Can you work these out from the drawing? Everything is in mm from the part's minimum corner. Coordinates: 2 decimals unless noted, no trailing zeros. Loops run counter-clockwise (first coordinate to the right, second up) from the corner with the lowest first, then second, coordinate; pieces in that order, holes last. Notation, with made-up numbers: M 76.5,58.5 L 102.5,58.5 A23 ccw 102.5,93.5 Z; hole C -24.75,-25 d10. An arc over 180 degrees is marked long. Write each question's results on one line, items separated by ' | '.
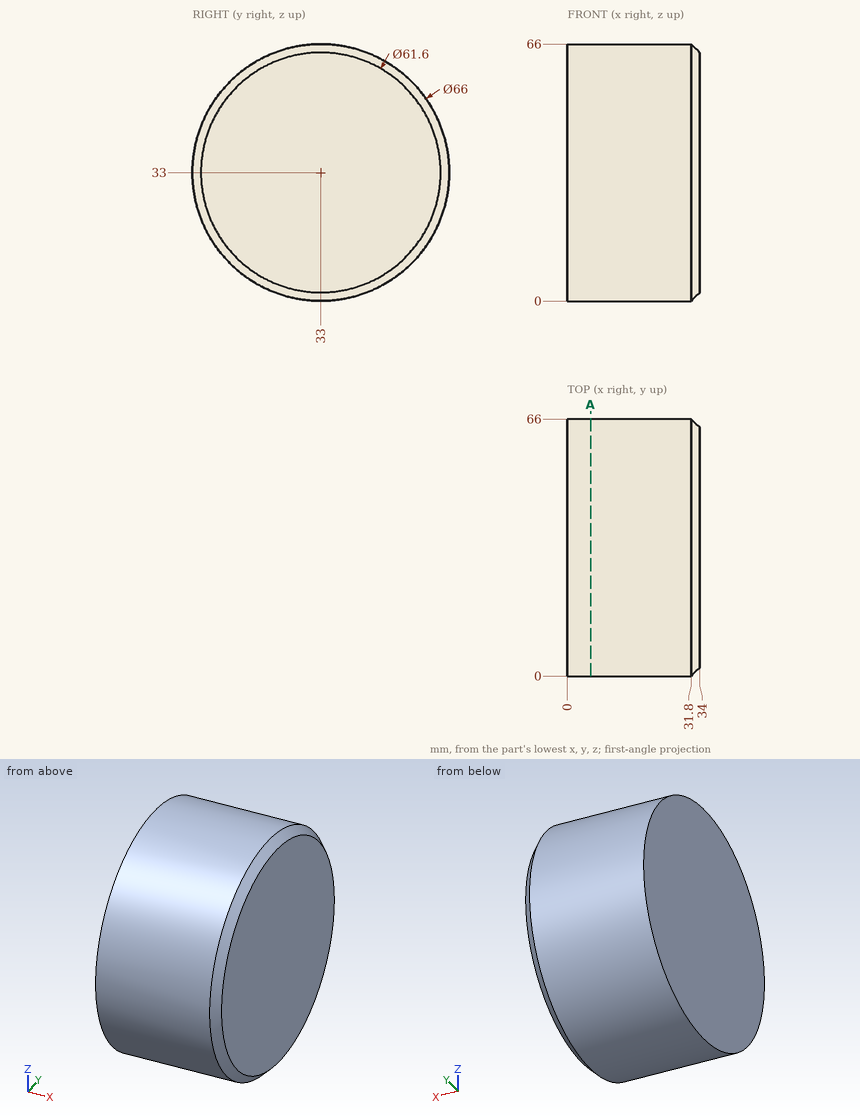
(1) Please list where these lines run through material, in increasing order: probe 1 along Z at (x, y) = (13, 34); probe 2 along Y at (x, z) = (11, 28.5). Write a range as from..to.
Reported:
probe 1: z = 0.02..65.98 | probe 2: y = 0.31..65.69
(2) Will these pins go through, and if not, where does the flat tip stop? P1, Ø10, axis at x = 9, z = 45, coming from the -Y side; P2, Ø10, axis at x = 30.5, z = 24, coming from the +Y side; P3, Ø1.5, axis at x = 22.5, y = 38.5, coming from the +Z side.
Reported:
P1: stops at y = 0.75 | P2: stops at y = 65.76 | P3: stops at z = 65.66
(3) Imagine slicing it at A-A, the plane x = 6. List the corners of the cut face in (y, z) for me.
Reported:
outline: C 33,33 d66
